Input: part model. Units: mm. Frame: model coordinates. Face numbers are marked on the shaded views. A direction names the side the tool comes from. Give positions to 0.01 mm unless a question says otherwise; leave off trailing zeros. Loops run counter-clockwise (first coordinate to the right, second up) from the corner with the lowest first, then second, coordinate; pieces in that order, holes last. Notation, with made-up numbers: M 41,27 L 69,27 A29 ccw 69,48 Z; hole C 72.25,77.5 d10. An arc over 180 degrees is marked long. Answer as a JSON object with one key per item and string values. Group by question number.
1) Section query B-B on z = -4. Return loops of the section in (x, y), plus the area to 3 significant figures.
2) Ray query, L1, parallel to Z at x = -4, y = -1.5; L2, parallel to X at y = 1.75, z = -8; L3, parallel to X at y = -8.25, z = 20.5. Return the intervals inside material, ascending.
3) First-contact query: P1, Ø1.9, axis at x = -5, z = 3, coming from the -Y side; P2, Ø6, axis at x = -20, y = -3.5, coming from the -Z side; P3, Ø3, axis at y = 0.5, z = 33.5, coming from the +X side. Flat tips, straight axial feed; report the tip coordinate or a pass-through.
4) Access query for the marked faces 4, 5 and 6. Directions: +Z, -Z, +X, -X, +Y, -Y. A direction counts if a zero-diameter tool reaches every point of the face in a straight line with its end or side. Return the directions, or none.
5) Draft query along Z for the marked faces 1, 2 and 3. Return one class per face: +Z half, -Z half, draft (parallel to the pull), parting line (faces both ways), or undercut.
6) Section query A-A on y = -6. Count the separate pieces of the cut face and the enclosed holes in it, plus the area to 3 significant figures.
7) Section query D-D on y = 2. Return loops of the section in (x, z).
8) Section query C-C on x = 17.5. Return loops of the section in (y, z), plus the area to 3 significant figures.
from build123d import *

# Parameters (mm, degrees)
VYSUNOUT_TENKOST_NN_1_DEPTH   = 9
VYSUNOUT_TENKOST_NN_2_DEPTH   = 7.5
VYSUNOUT_TENKOST_NN_2_2_DEPTH = 7.5
P_IDAT_VYSUNUT_M2_DEPTH       = 3
VYSUNOUT_START                = 3
VYSUNOUT_TENKOST_NN_3_DEPTH   = 3
SKICA4_R                      = 7.599478253
ODEBRAT_VYSUNUT_M1_DEPTH      = 10


with BuildPart() as part:
    # Skica3 → Vysunout tenkost_nn_1 (new body)
    with BuildSketch(Plane(origin=(0, 0, 0), x_dir=(1, 0, 0), z_dir=(0, 1, 0))):
        with BuildLine():
            ThreePointArc((13.318818193, -36.180678557), (16.919790609, -40.236611382), (21.547993361, -37.408655814))
            ThreePointArc((21.547993361, -37.408655814), (24.391270235, -18.641089057), (20.614348293, -0.038921281))
            ThreePointArc((20.614348293, -0.038921281), (20.561150024, 0.629518412), (20.890277717, 1.213741521))
            ThreePointArc((20.890277717, 1.213741521), (22.159844041, 18.012545588), (5.58094625, 21.004495587))
            ThreePointArc((5.58094625, 21.004495587), (0, 19.413874141), (-5.58094625, 21.004495587))
            ThreePointArc((-5.58094625, 21.004495587), (-22.159844041, 18.012545588), (-20.890277717, 1.213741521))
            ThreePointArc((-20.890277717, 1.213741521), (-20.561150024, 0.629518412), (-20.614348293, -0.038921281))
            ThreePointArc((-20.614348293, -0.038921281), (-24.391270235, -18.641089057), (-21.547993361, -37.408655814))
            ThreePointArc((-21.547993361, -37.408655814), (-16.919790609, -40.236611382), (-13.318818193, -36.180678557))
            Line((-13.318818193, -36.180678557), (-15.317951996, -36.121822462))
            ThreePointArc((-15.317951996, -36.121822462), (-17.214967104, -38.2585136), (-19.653133669, -36.768728669))
            ThreePointArc((-19.653133669, -36.768728669), (-22.391894143, -18.691041449), (-18.753808587, -0.772673285))
            ThreePointArc((-18.753808587, -0.772673285), (-18.607973584, 1.059752989), (-19.510227352, 2.661312241))
            ThreePointArc((-19.510227352, 2.661312241), (-20.577911445, 16.788826149), (-6.635335046, 19.305006173))
            ThreePointArc((-6.635335046, 19.305006173), (0, 17.413874141), (6.635335046, 19.305006173))
            ThreePointArc((6.635335046, 19.305006173), (20.577911445, 16.788826149), (19.510227352, 2.661312241))
            ThreePointArc((19.510227352, 2.661312241), (18.607973584, 1.059752989), (18.753808587, -0.772673285))
            ThreePointArc((18.753808587, -0.772673285), (22.391894143, -18.691041449), (19.653133669, -36.768728669))
            ThreePointArc((19.653133669, -36.768728669), (17.214967104, -38.2585136), (15.317951996, -36.121822462))
            Line((15.317951996, -36.121822462), (13.318818193, -36.180678557))
        make_face()
        with BuildLine():
            ThreePointArc((15.479480606, -36.942506696), (11.363736232, -25.348385806), (3.532419897, -15.859788681))
            ThreePointArc((3.532419897, -15.859788681), (0, -14.557634697), (-3.532419897, -15.859788681))
            ThreePointArc((-3.532419897, -15.859788681), (-11.363736232, -25.348385806), (-15.479480606, -36.942506696))
            Line((-15.479480606, -36.942506696), (-13.507192877, -37.274291437))
            ThreePointArc((-13.507192877, -37.274291437), (-9.623698487, -26.334422643), (-2.234300531, -17.38126366))
            ThreePointArc((-2.234300531, -17.38126366), (0, -16.557634697), (2.234300531, -17.38126366))
            ThreePointArc((2.234300531, -17.38126366), (9.623698487, -26.334422643), (13.507192877, -37.274291437))
            Line((13.507192877, -37.274291437), (15.479480606, -36.942506696))
        make_face()
    extrude(amount=-VYSUNOUT_TENKOST_NN_1_DEPTH)



with BuildPart() as body_2:
    # Skica3_3 → Vysunout tenkost_nn_2 (new body)
    with BuildSketch(Plane(origin=(0, 0, 0), x_dir=(1, 0, 0), z_dir=(0, 1, 0))):
        with BuildLine():
            ThreePointArc((-9.651511204, 20.15475088), (0.145367606, 16.213794321), (9.85696713, 20.360456559))
            Line((9.85696713, 20.360456559), (10.571915059, 19.661278857))
            ThreePointArc((10.571915059, 19.661278857), (0.155911444, 15.213849909), (-10.351556954, 19.440652884))
            Line((-10.351556954, 19.440652884), (-9.651511204, 20.15475088))
        make_face()
    extrude(amount=-VYSUNOUT_TENKOST_NN_2_DEPTH)


with BuildPart() as body_3:
    # Skica3_3 → Vysunout tenkost_nn_2 2 (new body)
    with BuildSketch(Plane(origin=(0, 0, 0), x_dir=(1, 0, 0), z_dir=(0, 1, 0))):
        with BuildLine():
            ThreePointArc((-14.318385094, -0.405797283), (-0.353145852, -5.812609189), (13.842408307, -1.043147566))
            Line((13.842408307, -1.043147566), (14.464095548, -1.82641315))
            ThreePointArc((14.464095548, -1.82641315), (-0.375772598, -6.812353171), (-14.974872193, -1.160134535))
            Line((-14.974872193, -1.160134535), (-14.318385094, -0.405797283))
        make_face()
    extrude(amount=-VYSUNOUT_TENKOST_NN_2_2_DEPTH)


with BuildPart() as part_1:
    add(part.part)

    add(body_2.part)  # P_idat vysunut_m2 merges body 2

    add(body_3.part)  # P_idat vysunut_m2 merges body 3
    # Skica3_4 → P_idat vysunut_m2 (add)
    with BuildSketch(Plane(origin=(0, 0, 0), x_dir=(1, 0, 0), z_dir=(0, 1, 0))):
        with BuildLine():
            ThreePointArc((6.108140648, 20.15475088), (0, 18.413874141), (-6.108140648, 20.15475088))
            ThreePointArc((-6.108140648, 20.15475088), (-21.368877743, 17.400685868), (-20.200252534, 1.937526881))
            ThreePointArc((-20.200252534, 1.937526881), (-19.584561804, 0.844635701), (-19.68407844, -0.405797283))
            ThreePointArc((-19.68407844, -0.405797283), (-23.391582189, -18.666065253), (-20.600563515, -37.088692241))
            ThreePointArc((-20.600563515, -37.088692241), (-17.553998549, -39.282880534), (-14.493336742, -37.108399066))
            ThreePointArc((-14.493336742, -37.108399066), (-10.493717359, -25.841404225), (-2.883360214, -16.620526171))
            ThreePointArc((-2.883360214, -16.620526171), (0, -15.557634697), (2.883360214, -16.620526171))
            ThreePointArc((2.883360214, -16.620526171), (10.493717359, -25.841404225), (14.493336742, -37.108399066))
            ThreePointArc((14.493336742, -37.108399066), (17.553998549, -39.282880534), (20.600563515, -37.088692241))
            ThreePointArc((20.600563515, -37.088692241), (23.391582189, -18.666065253), (19.68407844, -0.405797283))
            ThreePointArc((19.68407844, -0.405797283), (19.584561804, 0.844635701), (20.200252534, 1.937526881))
            ThreePointArc((20.200252534, 1.937526881), (21.368877743, 17.400685868), (6.108140648, 20.15475088))
        make_face()
    extrude(amount=P_IDAT_VYSUNUT_M2_DEPTH)

    # Skica3_5 → Vysunout tenkost_nn_3 (add)
    with BuildSketch(Plane(origin=(0, 0, 0), x_dir=(1, 0, 0), z_dir=(0, 1, 0)).offset(VYSUNOUT_START)):
        with BuildLine():
            ThreePointArc((13.318818193, -36.180678557), (16.919790609, -40.236611382), (21.547993361, -37.408655814))
            ThreePointArc((21.547993361, -37.408655814), (24.391270235, -18.641089057), (20.614348293, -0.038921281))
            ThreePointArc((20.614348293, -0.038921281), (20.561150024, 0.629518412), (20.890277717, 1.213741521))
            ThreePointArc((20.890277717, 1.213741521), (22.159844041, 18.012545588), (5.58094625, 21.004495587))
            ThreePointArc((5.58094625, 21.004495587), (0, 19.413874141), (-5.58094625, 21.004495587))
            ThreePointArc((-5.58094625, 21.004495587), (-22.159844041, 18.012545588), (-20.890277717, 1.213741521))
            ThreePointArc((-20.890277717, 1.213741521), (-20.561150024, 0.629518412), (-20.614348293, -0.038921281))
            ThreePointArc((-20.614348293, -0.038921281), (-24.391270235, -18.641089057), (-21.547993361, -37.408655814))
            ThreePointArc((-21.547993361, -37.408655814), (-16.919790609, -40.236611382), (-13.318818193, -36.180678557))
            Line((-13.318818193, -36.180678557), (-15.317951996, -36.121822462))
            ThreePointArc((-15.317951996, -36.121822462), (-17.214967104, -38.2585136), (-19.653133669, -36.768728669))
            ThreePointArc((-19.653133669, -36.768728669), (-22.391894143, -18.691041449), (-18.753808587, -0.772673285))
            ThreePointArc((-18.753808587, -0.772673285), (-18.607973584, 1.059752989), (-19.510227352, 2.661312241))
            ThreePointArc((-19.510227352, 2.661312241), (-20.577911445, 16.788826149), (-6.635335046, 19.305006173))
            ThreePointArc((-6.635335046, 19.305006173), (0, 17.413874141), (6.635335046, 19.305006173))
            ThreePointArc((6.635335046, 19.305006173), (20.577911445, 16.788826149), (19.510227352, 2.661312241))
            ThreePointArc((19.510227352, 2.661312241), (18.607973584, 1.059752989), (18.753808587, -0.772673285))
            ThreePointArc((18.753808587, -0.772673285), (22.391894143, -18.691041449), (19.653133669, -36.768728669))
            ThreePointArc((19.653133669, -36.768728669), (17.214967104, -38.2585136), (15.317951996, -36.121822462))
            Line((15.317951996, -36.121822462), (13.318818193, -36.180678557))
        make_face()
        with BuildLine():
            ThreePointArc((15.479480606, -36.942506696), (11.363736232, -25.348385806), (3.532419897, -15.859788681))
            ThreePointArc((3.532419897, -15.859788681), (0, -14.557634697), (-3.532419897, -15.859788681))
            ThreePointArc((-3.532419897, -15.859788681), (-11.363736232, -25.348385806), (-15.479480606, -36.942506696))
            Line((-15.479480606, -36.942506696), (-13.507192877, -37.274291437))
            ThreePointArc((-13.507192877, -37.274291437), (-9.623698487, -26.334422643), (-2.234300531, -17.38126366))
            ThreePointArc((-2.234300531, -17.38126366), (0, -16.557634697), (2.234300531, -17.38126366))
            ThreePointArc((2.234300531, -17.38126366), (9.623698487, -26.334422643), (13.507192877, -37.274291437))
            Line((13.507192877, -37.274291437), (15.479480606, -36.942506696))
        make_face()
        with BuildLine():
            ThreePointArc((-10.351556954, 19.440652884), (0.155911444, 15.213849909), (10.571915059, 19.661278857))
            Line((10.571915059, 19.661278857), (9.1420192, 21.05963426))
            ThreePointArc((9.1420192, 21.05963426), (0.134823768, 17.213738734), (-8.951465454, 20.868848876))
            Line((-8.951465454, 20.868848876), (-10.351556954, 19.440652884))
        make_face()
        with BuildLine():
            ThreePointArc((-14.974872193, -1.160134535), (-0.375772598, -6.812353171), (14.464095548, -1.82641315))
            Line((14.464095548, -1.82641315), (13.220721067, -0.259881982))
            ThreePointArc((13.220721067, -0.259881982), (-0.330519107, -4.812865207), (-13.661897996, 0.348539969))
            Line((-13.661897996, 0.348539969), (-14.974872193, -1.160134535))
        make_face()
    extrude(amount=-VYSUNOUT_TENKOST_NN_3_DEPTH)

    # Skica4 → Odebrat vysunut_m1 (cut)
    with BuildSketch(Plane(origin=(0, 0, 0), x_dir=(1, 0, 0), z_dir=(0, 1, 0))):
        with Locations(Location((-12.211626463, 10.317004534, 0), (0, 0, 270))):
            Circle(SKICA4_R)
        with Locations(Location((12.211626463, 10.317004534, 0), (0, 0, 270))):
            Circle(SKICA4_R)
    extrude(amount=ODEBRAT_VYSUNUT_M1_DEPTH, mode=Mode.SUBTRACT)


solid = part_1.part
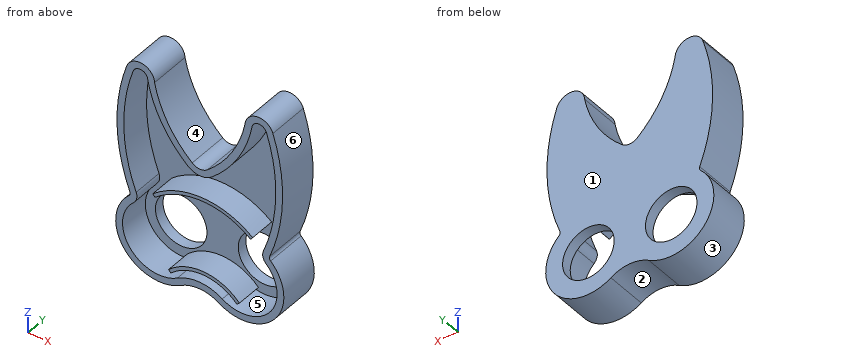
Output:
{
 "1": {"outline": "M -23.09,-9 L -20.7,-9 L -20.7,0 L -16.44,0 L -16.44,3 L -23.09,3 Z; M -7.99,0 L 7.99,0 L 7.99,3 L -7.99,3 Z; M 16.44,0 L 20.7,0 L 20.7,-9 L 23.09,-9 L 23.09,3 L 16.44,3 Z", "area": "131 mm^2"},
 "2": {"L1": "z = -20.2 to -18.07, -16.81 to -15.76, 5.42 to 6.44, 16.27 to 19", "L2": "x = -24.57 to -19.45, -4.97 to 4.97, 19.45 to 24.57", "L3": "x = -24.41 to -22.41, -8.06 to -5.43, 5.43 to 8.06, 22.41 to 24.41"},
 "3": {"P1": "stops at y = 0", "P2": "stops at z = -21.95", "P3": "stops at x = 23.07"},
 "4": {"face 4": "+Z, +Y, -Y", "face 5": "-Y", "face 6": "+X, +Y, -Y"},
 "5": {"face 1": "draft", "face 2": "-Z half", "face 3": "undercut"},
 "6": {"separate pieces": "3", "enclosed holes": "1", "area": "516 mm^2"},
 "7": {"outline": "M -21.55,37.41 A54.41 ccw -20.61,0.04 A1.15 cw -20.89,-1.21 A12.58 ccw -5.58,-21 A10.59 cw 5.58,-21 A12.58 ccw 20.89,-1.21 A1.15 cw 20.61,0.04 A54.41 ccw 21.55,37.41 A4.23 ccw 13.32,36.27 A33.44 cw 2.23,17.38 A3.44 cw -2.23,17.38 A33.44 cw -13.32,36.27 A4.23 ccw Z; hole C -12.21,-10.32 d15.2; hole C 12.21,-10.32 d15.2"},
 "8": {"outline": "M -9,-21.73 L 3,-21.73 L 3,-15.77 L 0,-15.77 L 0,-19.48 L -9,-19.48 Z; M -9,38.28 L 0,38.28 L 0,-4.86 L 3,-4.86 L 3,40.28 L -9,40.28 Z", "area": "192 mm^2"}
}
